Autodesk Inventor part; units mm, degrees
ref_plane "YZ Plane" through (0, 0, 0) normal (1, 0, 0) x (0, 1, 0)
ref_plane "XZ Plane" through (0, 0, 0) normal (0, 1, 0) x (-1, 0, 0)
ref_plane "XY Plane" through (0, 0, 0) normal (0, 0, 1) x (1, 0, 0)
sketch "スケッチ1" plane through (0, 0, 0) normal (0, 0, 1) x (1, 0, 0)
  circle A0 centre (0, 0) radius 9.75
  circle A1 centre (0, 0) radius 4.3
  dimension "d0" = 19.5
  dimension "d1" = 8.6
extrude "押し出し1" add sketch "スケッチ1" along normal blind 1
sketch "スケッチ2" plane through (0, 0, 1) normal (0, 0, 1) x (1, 0, 0)
  circle A0 centre (0, 0) radius 8
  point P0 (0, 8)
  point P1 (-8, 0)
  point P2 (0, -8)
  point P3 (8, 0)
  dimension "d4" = 16
  dimension "d7" = 360
hole "穴1" at (0, 8, 1) at (-8, 0, 1) at (0, -8, 1) at (8, 0, 1) direction (0, 0, -1) diameter 2.5 end through all
properties part number "rotor_shim"
CAD build for the part. Positions are in the model's coordinates, mm. Round coordinates to 2 decimals unless told otherwise and drop trailing zeros. Order: outer loops, then holes, each group sorted by start corner. A loop starts at its lowest first (then second) coordinate and runs counter-clockwise, first axis right, second up. Notation, with made-up numbers: (74, 10.25) - (131, 10.25) arc R19 cw to (131, 32.25) - close; hole circle Ø10 at (75.5, -36.5). An arc over 180 degrees is marked (long way). Answer as CSV lines item,"result". Start each with the question number.
1. Pull direction X, two halves, no side cores. Call faces 1 (the face through (4, -2, 0)), 2 (the face through (-6.78, 0.27, 0.49)), 3 (the face through (-1.269, -9.667, 0.493)): +X half, -X half, draft (parallel to the pull), parting line (faces both ways), or undercut.
2. Drill centre lines: L1, parallel to Y at x = 0, z = 0.55; L2, parallel to X at y = -1, z = 0.8; L3, parallel to X at y = 7, z = 0.25. Where is each one in solid material? Low to high. Write a range as [from, to].
3. Saw through at C-C, the plane x = -0.75. Write the cut outline in (y, z).
4. Saw through at B-B, the plane z = 0.65. Write the cut outline in (x, y).
5. Saw through at A-A, the plane y = 0. Write the cut outline in (x, z).
6. Saw through at D-D, the plane x = 8. Write the cut outline in (y, z).
7. Pin check, flat tip, straight feed: pin 1 (5 mm diameter, centred on x = 0, y = 0, fed in from +Z). Stop position of the tip, or through.
Model answer:
1,face 1,"draft"
1,face 2,"undercut"
1,face 3,"parting line"
2,L1,"y = [-9.75, -9.25], [-6.75, -4.3], [4.3, 6.75], [9.25, 9.75]"
2,L2,"x = [-9.7, -8.75], [-7.25, -4.18], [4.18, 7.25], [8.75, 9.7]"
2,L3,"x = [-6.79, -0.75], [0.75, 6.79]"
3,outline,"(-9.72, 0) - (-9, 0) - (-9, 1) - (-9.72, 1) - close; (-7, 0) - (-4.23, 0) - (-4.23, 1) - (-7, 1) - close; (4.23, 0) - (7, 0) - (7, 1) - (4.23, 1) - close; (9, 0) - (9.72, 0) - (9.72, 1) - (9, 1) - close"
4,outline,"circle Ø19.5 at (0, 0); hole circle Ø2.5 at (-8, 0); hole circle Ø8.6 at (0, 0); hole circle Ø2.5 at (0, -8); hole circle Ø2.5 at (0, 8); hole circle Ø2.5 at (8, 0)"
5,outline,"(-9.75, 0) - (-9.25, 0) - (-9.25, 1) - (-9.75, 1) - close; (-6.75, 0) - (-4.3, 0) - (-4.3, 1) - (-6.75, 1) - close; (4.3, 0) - (6.75, 0) - (6.75, 1) - (4.3, 1) - close; (9.25, 0) - (9.75, 0) - (9.75, 1) - (9.25, 1) - close"
6,outline,"(-5.57, 0) - (-1.25, 0) - (-1.25, 1) - (-5.57, 1) - close; (1.25, 0) - (5.57, 0) - (5.57, 1) - (1.25, 1) - close"
7,pin 1,"passes through"
